Check sheet for the modelled part. Datum: model origin and axes. Units: mm. A direction names the side the tool comes from. Coordinates: 2 decimals unless noted, no trailing zeros. Loops run counter-clockwise (first coordinate to the right, second up) from the corner with the lowest first, then second, coordinate; pieces in that order, holes last. Notation, with made-up numbers: M 67,80 L 119,80 A15 cw 119,91 Z; hole C 7.5,76 d4. An arc over 180 degrees is marked long. Write each question's results on one line, items separated by ' | '. Start each with the question number.
from build123d import *

# Parameters (mm, degrees)
SKETCH1_R           = 9.48
BOSS_EXTRUDE1_DEPTH = 5
SKETCH2_R           = 2
CUT_EXTRUDE1_DEPTH  = 3


with BuildPart() as part:
    # Sketch1 → Boss-Extrude1 (new body)
    with BuildSketch(Plane(origin=(0, 0, 0), x_dir=(1, 0, 0), z_dir=(0, 1, 0))):
        with Locations(Location((0, 0, 0), (0, 0, 270))):
            Circle(SKETCH1_R)
    extrude(amount=-BOSS_EXTRUDE1_DEPTH)

    # Sketch2 → Cut-Extrude1 (cut)
    with BuildSketch(Plane(origin=(0, 0, 0), x_dir=(1, 0, 0), z_dir=(0, 1, 0))):
        with Locations(Location((3.329285114, 4.894478506, 0), (0, 0, 270))):
            Circle(SKETCH2_R)
        with Locations(Location((3.329285114, -4.894478506, 0), (0, 0, 90))):
            Circle(SKETCH2_R)
    extrude(amount=-CUT_EXTRUDE1_DEPTH, mode=Mode.SUBTRACT)


solid = part.part
Item 1: Depth check by flat-ended pin: P1, Ø2.5, axis at x = 3.33, z = 4.89, coming from the +Y side; P2, Ø8, axis at x = 7.5, z = 0, coming from the +Y side; P3, Ø3, axis at y = -3, z = 4.5, coming from the +X side. Enter the tip coordinate at first touch or a pass-through.
Item 2: Section check A-A (z = -3.5). Record the cut outline in (x, y).
Item 3: Tool access check on faces 4 (the face through (0, 0, 0)), 5 (the face through (3, -3, -5)). Record the directions out of +Z, -Z, +X, -X, +Y, -Y that give a thin tool (end or side, any length) a straight path to the whole face; none if there is none.
Item 4: Section check B-B (x = 2.5). Record the cut outline in (y, z), plus the area to 3 significant figures.
Item 5: Release check for a two-part mould opening along Z. For faces 1 (the face through (2.85, -2.46, 9.04)), 2 (the face through (0, -5, 0)), 3 (the face through (3.93, -1.479, -2.987)) record: +Z half, -Z half, draft (parallel to the pull), parting line (faces both ways), or undercut.
Item 6: Section check C-C (y = -2.7). Record the cut outline in (x, z), plus the area to 3 significant figures.
Item 7: Section check D-D (z = -6.5). Record the cut outline in (x, y), plus the area to 3 significant figures.
Item 8: Thickness scan on line 1 (Z direction, x = 4.75, y = -1.25); line 2 (Z direction, x = 2.5, y = -2.9); line 3 (X direction, y = -1.6, z = 0). Record the ranges inside material, lowest first.
Computed values:
1) P1: stops at y = -3 | P2: stops at y = 0 | P3: stops at x = 8.99
2) outline: M -8.81,-5 L 8.81,-5 L 8.81,0 L 4.76,0 L 4.76,-3 L 1.9,-3 L 1.9,0 L -8.81,0 Z
3) face 4: +Z, -Z, +X, -X, +Y | face 5: +Y
4) outline: M -5,-9.14 L 0,-9.14 L 0,-6.71 L -3,-6.71 L -3,-3.07 L 0,-3.07 L 0,3.07 L -3,3.07 L -3,6.71 L 0,6.71 L 0,9.14 L -5,9.14 Z | area: 69.6 mm²
5) face 1: parting line | face 2: draft | face 3: undercut
6) outline: C 0,0 d18.96; hole C 3.33,-4.89 d4; hole C 3.33,4.89 d4 | area: 257 mm²
7) outline: M -6.9,-5 L 6.9,-5 L 6.9,0 L 4.52,0 L 4.52,-3 L 2.14,-3 L 2.14,0 L -6.9,0 Z | area: 61.9 mm²
8) line 1: z = -8.2 to -6.3, -3.49 to 3.49, 6.3 to 8.2 | line 2: z = -9.14 to -6.71, -3.07 to 3.07, 6.71 to 9.14 | line 3: x = -9.48 to 9.48
